```python
from build123d import *

# Parameters (mm, degrees)
F1_DEPTH = 25


with BuildPart() as f1:
    # F0 (on Front) → F1 (new body)
    with BuildSketch(Plane.XZ):
        with BuildLine():
            Line((-59.432037, 80), (-129.432037, 80))
            Line((-129.432037, 80), (-129.432037, 30))
            ThreePointArc((-129.432037, 30), (-159.432037, 0), (-129.432037, -30))
            Line((-129.432037, -30), (-129.432037, -80))
            Line((-129.432037, -80), (-59.432037, -80))
            ThreePointArc((-59.432037, -80), (0, -99.660258), (59.432037, -80))
            Line((59.432037, -80), (129.432037, -80))
            Line((129.432037, -80), (129.432037, -30))
            ThreePointArc((129.432037, -30), (159.432037, 0), (129.432037, 30))
            Line((129.432037, 30), (129.432037, 80))
            Line((129.432037, 80), (59.432037, 80))
            ThreePointArc((59.432037, 80), (0, 99.660258), (-59.432037, 80))
        make_face()
        with BuildLine():
            Line((84.432037, -52.494368), (84.432037, 0))
            Line((84.432037, 0), (84.432037, 52.154386))
            ThreePointArc((84.432037, 52.154386), (87.36097, 59.225454), (94.432037, 62.154386))
            Line((94.432037, 62.154386), (104.432037, 62.154386))
            ThreePointArc((104.432037, 62.154386), (111.503105, 59.225454), (114.432037, 52.154386))
            Line((114.432037, 52.154386), (114.432037, -52.494368))
            ThreePointArc((114.432037, -52.494368), (111.503105, -59.565436), (104.432037, -62.494368))
            Line((104.432037, -62.494368), (94.432037, -62.494368))
            ThreePointArc((94.432037, -62.494368), (87.36097, -59.565436), (84.432037, -52.494368))
        make_face(mode=Mode.SUBTRACT)
        with BuildLine():
            Line((-84.432037, 55), (-84.432037, 0))
            Line((-84.432037, 0), (-84.432037, -55))
            ThreePointArc((-84.432037, -55), (-87.36097, -62.071068), (-94.432037, -65))
            Line((-94.432037, -65), (-104.432037, -65))
            ThreePointArc((-104.432037, -65), (-111.503105, -62.071068), (-114.432037, -55))
            Line((-114.432037, -55), (-114.432037, 55))
            ThreePointArc((-114.432037, 55), (-111.503105, 62.071068), (-104.432037, 65))
            Line((-104.432037, 65), (-94.432037, 65))
            ThreePointArc((-94.432037, 65), (-87.36097, 62.071068), (-84.432037, 55))
        make_face(mode=Mode.SUBTRACT)
        with BuildLine():
            ThreePointArc((0, 60), (42.426407, 42.426407), (60, 0))
            ThreePointArc((60, 0), (0, -60), (-60, 0))
            ThreePointArc((-60, 0), (-42.426407, 42.426407), (0, 60))
        make_face(mode=Mode.SUBTRACT)
    extrude(amount=F1_DEPTH)


solid = f1.part
```
Source: CAD feature listing. Evaluate the final solid. Frame: model axes, mm. A direction names the side the tool comes from. Coordinates: 2 decimals unless noted, no trailing zeros. Write each loop counter-clockwise with the first axis right and the second up, starting at its lowest first coordinate (ties: lowest second). Pieces come first, ordered by that corner, then holes. Notation, with made-up numbers: (8, 18) - (35, 18) arc R23 ccw to (35, 45) - close; hole circle Ø9 at (84.5, 62.5). An arc over 180 degrees is marked (long way). Answer as a JSON object with one key per item and string values.
Q1. First-contact query: pin 1 Ø12.5 at (y, z) = (-7.5, 56.5) entering from +X; pin 2 Ø8 at (x, y) = (-125, -18) entering from -Z; pin 3 Ø12.5 at (y, z) = (-9, -18.5) entering from +X. Flat tips, straight axial feed; report the tip coordinate or a pass-through.
Ans:
{"pin 1": "stops at x = 129.43", "pin 2": "stops at z = -80", "pin 3": "stops at x = 156.82"}
Q2. Section query A-A, the plane x = -15. Output: boundary loops of the cut face in (y, z).
Ans:
{"outline": "(-25, -98.52) - (0, -98.52) - (0, -58.09) - (-25, -58.09) - close; (-25, 58.09) - (0, 58.09) - (0, 98.52) - (-25, 98.52) - close"}
Q3. Section query C-C, the plane z = -15. Output: boundary loops of the cut face in (x, y).
Ans:
{"outline": "(-155.41, -25) - (-114.43, -25) - (-114.43, 0) - (-155.41, 0) - close; (-84.43, -25) - (-58.09, -25) - (-58.09, 0) - (-84.43, 0) - close; (58.09, -25) - (84.43, -25) - (84.43, 0) - (58.09, 0) - close; (114.43, -25) - (155.41, -25) - (155.41, 0) - (114.43, 0) - close"}
Q4. Section query D-D, the plane z = -39. Output: boundary loops of the cut face in (x, y).
Ans:
{"outline": "(-129.43, -25) - (-114.43, -25) - (-114.43, 0) - (-129.43, 0) - close; (-84.43, -25) - (-45.6, -25) - (-45.6, 0) - (-84.43, 0) - close; (45.6, -25) - (84.43, -25) - (84.43, 0) - (45.6, 0) - close; (114.43, -25) - (129.43, -25) - (129.43, 0) - (114.43, 0) - close"}
Q5. Material intervals for line 1 (Z direction, x = 0, y = -8); line 2 (X direction, y = -8, z = 20); line 3 (X direction, y = -21, z = -32), sorted ascending. Write a range as [from, to].
Ans:
{"line 1": "z = [-99.66, -60], [60, 99.66]", "line 2": "x = [-151.79, -114.43], [-84.43, -56.57], [56.57, 84.43], [114.43, 151.79]", "line 3": "x = [-129.43, -114.43], [-84.43, -50.75], [50.75, 84.43], [114.43, 129.43]"}
Q6. Section query B-B, the plane y = -4. State how many separate pieces and enclosed holes the cut face has, plus the area to 3 significant figures.
Ans:
{"separate pieces": "1", "enclosed holes": "3", "area": "28,700 mm2"}
Q7. Draft query along X for faces 4 (the cylindrical face through (-87.44, -12.32, 62.15)), 5 (the cylindrical face through (87.284, -12.325, 59.147)), 6 (the cylindrical face through (-0.891, -12.325, -99.656)), 7 (the flat face through (129.432, -12, 55)). Return one class per face: released by +X, released by -X, zero draft, split by the parting line, or undercut.
Ans:
{"face 4": "undercut", "face 5": "undercut", "face 6": "split by the parting line", "face 7": "released by +X"}
Q8. Set-up query: faces 1 (the flat face through (-129.432, -12, -55)), 2 (the flat face through (129.432, -12, -55)), 3 (the cylindrical face through (111.425, -12.325, 59.303)). Return all of +Z, -Z, +X, -X, +Y, -Y with unobstructed straight access to the full face (end or side cutting, diameter ignored); none if empty.
Ans:
{"face 1": "-Z, -X, +Y, -Y", "face 2": "-Z, +X, +Y, -Y", "face 3": "+Y, -Y"}
